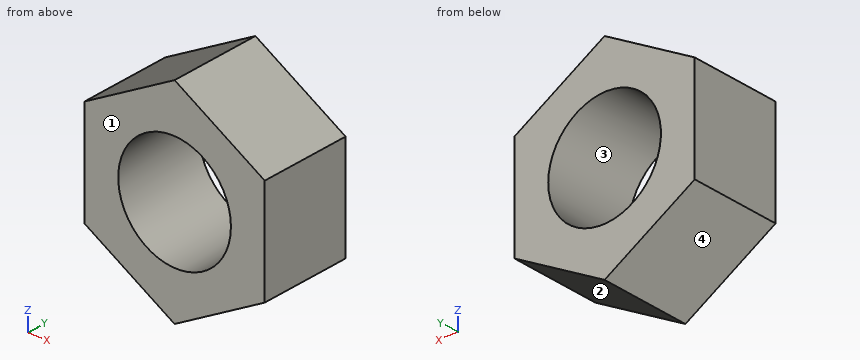
Solid Edge part; units mm, degrees
sketch "Sketch1" plane through (0, 0, 0) normal (0, -1, 0) x (1, 0, 0)
  line L0 (4, 2.3094) -> (0, 4.6188)
  line L1 (0, 4.6188) -> (-4, 2.3094)
  line L2 (-4, 2.3094) -> (-4, -2.3094)
  line L3 (-4, -2.3094) -> (0, -4.6188)
  line L4 (0, -4.6188) -> (4, -2.3094)
  line L5 (4, -2.3094) -> (4, 2.3094)
  circle A0 centre (0, 0) radius 2.5
extrude "Protrusion1" add sketch "Sketch1" against normal blind 4
cosmetic_thread "Thread1"
Part model, mm, in its own coordinate system. Face numbers are marked on the shaded views. Round coordinates to 2 decimals unless told otherwise and drop trailing zeros. Loops run counter-clockwise (first coordinate to the right, second up) from the corner with the lowest first, then second, coordinate; pieces in that order, holes last. Notation, with made-up numbers: (15.5, 40) -> (38.5, 40) arc R27 ccw to (38.5, 57) -> close; hole circle Ø11 at (13.5, 89). An arc over 180 degrees is marked (long way). Use a Markdown table: item, result.
1) Cut at A-A, the plane z = 1.5. List the corners of the cut face in (x, y), and give its area (3 significant figures).
The answers:
| item | result |
|---|---|
| outline | (-4, 0) -> (-2, 0) -> (-2, 4) -> (-4, 4) -> close; (2, 0) -> (4, 0) -> (4, 4) -> (2, 4) -> close |
| area | 16.0 mm2 |
2) Cut at C-C, the plane y = 0.3. List the corners of the cut face in (x, z).
The answers:
| item | result |
|---|---|
| outline | (-4, -2.31) -> (0, -4.62) -> (4, -2.31) -> (4, 2.31) -> (0, 4.62) -> (-4, 2.31) -> close; hole circle Ø5 at (0, 0) |
3) Cut at B-B, the plane x = 2. List the corners of the cut face in (y, z), and give its area (3 significant figures).
The answers:
| item | result |
|---|---|
| outline | (0, -3.46) -> (4, -3.46) -> (4, -1.5) -> (0, -1.5) -> close; (0, 1.5) -> (4, 1.5) -> (4, 3.46) -> (0, 3.46) -> close |
| area | 15.7 mm2 |
4) Pull direction X, two halves, no side cores. Call the marked faces 1, 2, 3 and 4: pulls with the +X half, pulls with the -X half, needs draft (parallel to the pull), parting line crosses it, or undercut.
The answers:
| item | result |
|---|---|
| face 1 | needs draft |
| face 2 | pulls with the +X half |
| face 3 | undercut |
| face 4 | pulls with the -X half |
5) Drop flat-ended pins along their axis: pin 1 Ø1.5 at (x, y) = (1.5, 2) entering from -Z; pin 2 Ø2 at (x, y) = (-0.5, 1) entering from -Z; pin 3 Ø4.5 at (x, z) = (0, 0) entering from -Y; pin 4 Ø1 at (x, y) = (-2.5, 2.5) entering from +Z. Give the stop position or say it passes through.
The answers:
| item | result |
|---|---|
| pin 1 | stops at z = -4.19 |
| pin 2 | stops at z = -4.62 |
| pin 3 | passes through |
| pin 4 | stops at z = 3.46 |
6) Probe line 1 (X direction, y = 1.6, z = -0.5); line 2 (Z direction, x = 2, y = 3.55); line 3 (Z direction, x = -0.5, y = 3.05). List the from-to ranges inside material, lowest first. Write a range as [from, to].
The answers:
| item | result |
|---|---|
| line 1 | x = [-4, -2.45], [2.45, 4] |
| line 2 | z = [-3.46, -1.5], [1.5, 3.46] |
| line 3 | z = [-4.33, -2.45], [2.45, 4.33] |
